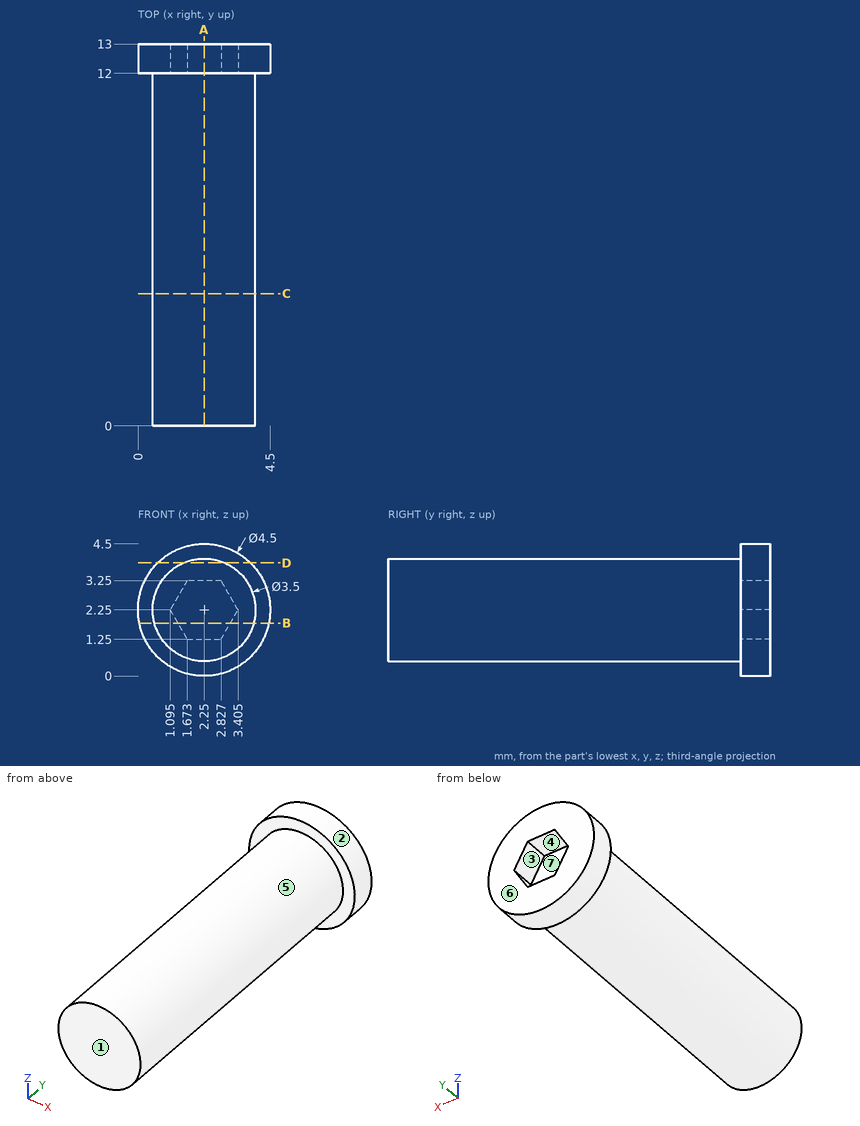
Answer from the drawing. Dimensions are ordinates in mm from the lowest x, y and z of the part. A direction names the side the tool comes from. Round coordinates to 2 decimals unless told otherwise and drop trailing zeros. Loops run counter-clockwise (first coordinate to the right, second up) from the corner with the lowest first, then second, coordinate; pieces in that order, holes last.
Q1. Section C-C on y = 4.5 is taken. Write down the section's boundary in (x, z).
Q2. Section D-D on z = 3.85 is taken. Write down the section's boundary in (x, y).
Q3. Which of the six approach directions +Z, -Z, +X, -X, +Y, -Y give full straight-line access (tool end or side, diameter ignored) to the marked faces 5, 6 and 7?
Q4. Determine the mould class of the marked faces 1, 2, 3 and 4 for opening direction Z: released by +Z, released by -Z, zero draft, split by the parting line, or undercut.
Q5. Each of these flat-tipped pins is pushed along its axis until it touches: pin 1 (1 mm diameter, centred on x = 2, y = 9.5, fed in from -Z); pin 2 (1.5 mm diameter, centred on y = 11.5, z = 1.5, fed in from -X); pin 3 (2 mm diameter, centred on y = 7, z = 1.5, fed in from -X). Where does it stop, or does it pass through?
Q6. Consider probe 1 along X at (y, z) = (9, 2.3); probe 2 along Y at (x, z) = (2.7, 2.25); probe 3 along Y at (x, z) = (0.95, 3.65). Determine where each line is inside the solid, lowest interval first.
Q7. Section A-A on x = 2.25 is taken. Write down the section's boundary in (y, z).
Q8. Section B-B on z = 1.8 is taken. Write down the section's boundary in (x, y) (1 decimal), and give its area (3 significant figures).
Output:
1. outline: circle Ø3.5 at (2.25, 2.25)
2. outline: (0.67, 12) - (1.54, 12) - (1.54, 0) - (2.96, 0) - (2.96, 12) - (3.83, 12) - (3.83, 13) - (0.67, 13) - close
3. face 5: -Y
3. face 6: +Z, -Z, +X, -X, +Y
3. face 7: +Y
4. face 1: zero draft
4. face 2: split by the parting line
4. face 3: undercut
4. face 4: undercut
5. pin 1: stops at z = 0.5
5. pin 2: stops at x = 0.01
5. pin 3: stops at x = 0.5
6. probe 1: x = 0.5 to 4
6. probe 2: y = 0 to 12
6. probe 3: y = 12 to 13
7. outline: (0, 0.5) - (12, 0.5) - (12, 0) - (13, 0) - (13, 1.25) - (12, 1.25) - (12, 3.25) - (13, 3.25) - (13, 4.5) - (12, 4.5) - (12, 4) - (0, 4) - close
8. outline: (0, 12) - (0.6, 12) - (0.6, 0) - (3.9, 0) - (3.9, 12) - (4.5, 12) - (4.5, 13) - (3.1, 13) - (3.1, 12) - (1.4, 12) - (1.4, 13) - (0, 13) - close
8. area: 43.2 mm2
